The model under review builds one solid part; all positions refer to its coordinate system, in mm. A direction names the side the tool comes from. Give positions to 0.01 mm unless a question says otherwise; leave off trailing zeros. Loops run counter-clockwise (first coordinate to the right, second up) from the corner with the lowest first, then second, coordinate; pieces in that order, holes last. Notation, with made-up numbers: (4, -20) -> (55, -20) arc R32 ccw to (55, 6) -> close; hole circle Ø6 at (53.5, 35). An arc over 180 degrees is marked (long way). Write each question's results on one line, items separated by ' | '. Start each with the question number.
Q1. Machinability: for faces 1 (the face through (-10, 4.107, 51)), 2 (the face through (16, 11.473, 3)), 3 (the face through (-16.571, -32, 6)), 4 (the face through (-11, -68.127, 6)), 5 (the face through (-10, 16.855, 55)), which of the approach directions +Z, -Z, +X, -X, +Y, -Y give a long, thin tool a straight path to every point of the face, cutting with its end or side? Answer none if there is none.
Q2. We need section C-C (z = 18). Write out the cut boundary in (x, y).
Q3. Wall thickness on L1, parallel to X at y = 6.5, z = 99.5; L2, parallel to Z at x = -10.5, y = -59.5; L3, parallel to Y at x = -12, z = 53: over which ranges is each line inside the solid? List them lowest first. Write a range as [from, to].
Q4. We need section B-B (y = -62). Write out the cut boundary in (x, z), plus the area to 3 significant figures.
Q5. We need section A-A (x = -11). Write out the cut boundary in (y, z), plus the area to 3 significant figures.
Q6. Insertion check: pin 1 Ø3.5 at (x, z) = (-9, 33) entering from -Y; pin 2 Ø3.5 at (x, z) = (-9, 34) entering from +Y; pin 3 Ø6.5 at (y, z) = (-17, 7) entering from +X; pin 4 Ø10 at (x, y) = (-24, -23) entering from +Z (3 decimals). Each pin has a flat end and moves straight along its axis. Give the tip position at first contact, or say it passes through.
from build123d import *

# Parameters (mm, degrees)
F0_W     = 11.8974833749
F0_H     = 12.7473026514
F1_DEPTH = 104
F2_W     = 12.1807525866
F2_H     = 72.517989669
F3_DEPTH = 13
F4_W     = 40
F4_H     = 5.6654671207
F5_DEPTH = 7
F6_DEPTH = 12.1
F7_DEPTH = 3


with BuildPart() as f1:
    # F0 (on Top) → F1 (new body)
    with BuildSketch(Plane.XY):
        with Locations((-10.339479195, 10.4811154306)):
            Rectangle(F0_W, F0_H)
    extrude(amount=F1_DEPTH)

    # F2 (on Top) → F3 (join)
    with BuildSketch(Plane.XY):
        with Locations((-10.4811156634, -31.868257327)):
            Rectangle(F2_W, F2_H)
    extrude(amount=F3_DEPTH)



with BuildPart() as f5:
    # F4 (on Top) → F5 (new body)
    with BuildSketch(Plane.XY):
        with Locations((15.8340851963, 14.3053061329)):
            Rectangle(F4_W, F4_H)
    extrude(amount=F5_DEPTH)


with BuildPart() as f5b:
    # F4 (on Top) → F5, piece 2 (new body)
    with BuildSketch(Plane.XY):
        with Locations((-36.5130412579, 14.3053061329)):
            Rectangle(F4_W, F4_H)
    extrude(amount=F5_DEPTH)


with BuildPart() as f1_1:
    add(f1.part)
    # F6 (add): a face of the model
    f6_faces = [f5b.part.faces().sort_by_distance(p)[0] for p in [
        (-16.5130412579, 14.3053061329, 3.5),
    ]]

    add(f5b.part)  # F6 merges F5b
    extrude(f6_faces, amount=F6_DEPTH)

    # F7 (add): a face of the model
    f7_faces = [f5.part.faces().sort_by_distance(p)[0] for p in [
        (-4.1659148037, 14.3053061329, 3.5),
    ]]

    add(f5.part)  # F7 merges F5
    extrude(f7_faces, amount=F7_DEPTH)


solid = f1_1.part
Output:
1) face 1: +Z, +X, -X, -Y | face 2: +Z, -Z, +X, -Y | face 3: +Z, -Z, -X, -Y | face 4: +Z, -Z, +X, -X, -Y | face 5: +Z, +X, -X, +Y
2) outline: (-16.29, 4.11) -> (-4.39, 4.11) -> (-4.39, 16.85) -> (-16.29, 16.85) -> close
3) L1: [-16.29, -4.39] | L2: [0, 13] | L3: [4.11, 16.85]
4) outline: (-16.57, 0) -> (-4.39, 0) -> (-4.39, 13) -> (-16.57, 13) -> close | area: 158 mm2
5) outline: (-68.13, 0) -> (17.14, 0) -> (17.14, 7) -> (16.85, 7) -> (16.85, 104) -> (4.11, 104) -> (4.11, 13) -> (-68.13, 13) -> close | area: 2,270 mm2
6) pin 1: y = 4.11 | pin 2: y = 16.85 | pin 3: x = -4.39 | pin 4: through
